```python
from build123d import *

# Parameters (mm, degrees)
SKETCH1_W           = 149
SKETCH1_H           = 168
SKETCH1_W_2         = 125
SKETCH1_H_2         = 144
BOSS_EXTRUDE1_DEPTH = 7
FILLET1_R           = 5
FILLET2_R           = 5
FILLET3_R           = 5
FILLET4_R           = 5
CUT_EXTRUDE1_DEPTH  = 3
SKETCH6_R           = 1.325
CUT_EXTRUDE2_DEPTH  = 4
CUT_EXTRUDE3_DEPTH  = 2


with BuildPart() as part:
    # Sketch1 → Boss-Extrude1 (new body)
    with BuildSketch(Plane(origin=(0, 0, 0), x_dir=(1, 0, 0), z_dir=(0, 1, 0))):
        with Locations((-8.812010444, -5.018276762)):
            Rectangle(SKETCH1_W, SKETCH1_H)
        with Locations((-8.812010444, -5.018276762)):
            Rectangle(SKETCH1_W_2, SKETCH1_H_2, mode=Mode.SUBTRACT)
    extrude(amount=BOSS_EXTRUDE1_DEPTH)

    # Fillet1
    fillet1_edges = [part.edges().sort_by_distance(p)[0] for p in [
        (65.687989556, 3.5, 89.018276762),
    ]]
    fillet(fillet1_edges, radius=FILLET1_R)

    # Fillet2
    fillet2_edges = [part.edges().sort_by_distance(p)[0] for p in [
        (-83.312010444, 3.5, 89.018276762),
    ]]
    fillet(fillet2_edges, radius=FILLET2_R)

    # Fillet3
    fillet3_edges = [part.edges().sort_by_distance(p)[0] for p in [
        (-83.312010444, 3.5, -78.981723238),
    ]]
    fillet(fillet3_edges, radius=FILLET3_R)

    # Fillet4
    fillet4_edges = [part.edges().sort_by_distance(p)[0] for p in [
        (65.687989556, 3.5, -78.981723238),
    ]]
    fillet(fillet4_edges, radius=FILLET4_R)

    # Sketch4 → Cut-Extrude1 (cut)
    with BuildSketch(Plane.XZ):
        Polygon((-40.312010444, 80.018276762), (-25.812010444, 80.018276762), (-25.812010444, 84.518276762), (-60.812010444, 84.518276762), (-60.812010444, 80.018276762), (-46.312010444, 80.018276762), (-46.312010444, 77.018276762), (-40.312010444, 77.018276762), align=None)
        Polygon((22.687989556, 77.018276762), (22.687989556, 80.018276762), (8.187989556, 80.018276762), (8.187989556, 84.518276762), (43.187989556, 84.518276762), (43.187989556, 80.018276762), (28.687989556, 80.018276762), (28.687989556, 77.018276762), align=None)
        Polygon((53.687989556, 47.018276762), (56.687989556, 47.018276762), (56.687989556, 66.518276762), (61.187989556, 66.518276762), (61.187989556, 21.518276762), (56.687989556, 21.518276762), (56.687989556, 41.018276762), (53.687989556, 41.018276762), align=None)
        Polygon((53.687989556, -35.981723238), (56.687989556, -35.981723238), (56.687989556, -13.981723238), (61.187989556, -13.981723238), (61.187989556, -63.981723238), (56.687989556, -63.981723238), (56.687989556, -41.981723238), (53.687989556, -41.981723238), align=None)
        Polygon((43.187989556, -69.981723238), (43.187989556, -74.481723238), (8.187989556, -74.481723238), (8.187989556, -69.981723238), (22.687989556, -69.981723238), (22.687989556, -66.981723238), (28.687989556, -66.981723238), (28.687989556, -69.981723238), align=None)
        Polygon((-40.312010444, -66.981723238), (-40.312010444, -69.981723238), (-25.812010444, -69.981723238), (-25.812010444, -74.481723238), (-60.812010444, -74.481723238), (-60.812010444, -69.981723238), (-46.312010444, -69.981723238), (-46.312010444, -66.981723238), align=None)
        Polygon((-71.312010444, -41.981723238), (-74.312010444, -41.981723238), (-74.312010444, -63.981723238), (-78.812010444, -63.981723238), (-78.812010444, -13.981723238), (-74.312010444, -13.981723238), (-74.312010444, -35.981723238), (-71.312010444, -35.981723238), align=None)
        Polygon((-71.312010444, 41.018276762), (-74.312010444, 41.018276762), (-74.312010444, 21.518276762), (-78.812010444, 21.518276762), (-78.812010444, 66.518276762), (-74.312010444, 66.518276762), (-74.312010444, 47.018276762), (-71.312010444, 47.018276762), align=None)
    extrude(amount=-CUT_EXTRUDE1_DEPTH, mode=Mode.SUBTRACT)

    # Sketch6 → Cut-Extrude2 (cut)
    with BuildSketch(Plane.XZ):
        with Locations(Location((-76.579777397, 82.286043715, 0), (0, 0, 270))):
            Circle(SKETCH6_R)
        with Locations(Location((58.955756509, 82.286043715, 0), (0, 0, 270))):
            Circle(SKETCH6_R)
        with Locations(Location((58.955756509, -72.249490191, 0), (0, 0, 270))):
            Circle(SKETCH6_R)
        with Locations(Location((-76.579777397, -72.249490191, 0), (0, 0, 270))):
            Circle(SKETCH6_R)
    extrude(amount=-CUT_EXTRUDE2_DEPTH, mode=Mode.SUBTRACT)

    # Sketch7 → Cut-Extrude3 (cut)
    with BuildSketch(Plane.XZ.offset(-3)):
        Polygon((53.687989556, -35.981723238), (56.687989556, -35.981723238), (56.687989556, -30.981723238), (61.187989556, -30.981723238), (61.187989556, -46.981723238), (56.687989556, -46.981723238), (56.687989556, -41.981723238), (53.687989556, -41.981723238), align=None)
        Polygon((53.687989556, 47.018276762), (56.687989556, 47.018276762), (56.687989556, 52.018276762), (61.187989556, 52.018276762), (61.187989556, 36.018276762), (56.687989556, 36.018276762), (56.687989556, 41.018276762), (53.687989556, 41.018276762), align=None)
        Polygon((28.687989556, 77.018276762), (28.687989556, 80.018276762), (33.687989556, 80.018276762), (33.687989556, 84.518276762), (17.687989556, 84.518276762), (17.687989556, 80.018276762), (22.687989556, 80.018276762), (22.687989556, 77.018276762), align=None)
        Polygon((-40.312010444, 77.018276762), (-40.312010444, 80.018276762), (-35.312010444, 80.018276762), (-35.312010444, 84.518276762), (-51.312010444, 84.518276762), (-51.312010444, 80.018276762), (-46.312010444, 80.018276762), (-46.312010444, 77.018276762), align=None)
        Polygon((-71.312010444, 47.018276762), (-74.312010444, 47.018276762), (-74.312010444, 52.018276762), (-78.812010444, 52.018276762), (-78.812010444, 36.018276762), (-74.312010444, 36.018276762), (-74.312010444, 41.018276762), (-71.312010444, 41.018276762), align=None)
        Polygon((-71.312010444, -35.981723238), (-74.312010444, -35.981723238), (-74.312010444, -30.981723238), (-78.812010444, -30.981723238), (-78.812010444, -46.981723238), (-74.312010444, -46.981723238), (-74.312010444, -41.981723238), (-71.312010444, -41.981723238), align=None)
        Polygon((-46.312010444, -66.981723238), (-46.312010444, -69.981723238), (-51.312010444, -69.981723238), (-51.312010444, -74.481723238), (-35.312010444, -74.481723238), (-35.312010444, -69.981723238), (-40.312010444, -69.981723238), (-40.312010444, -66.981723238), align=None)
        Polygon((22.687989556, -66.981723238), (22.687989556, -69.981723238), (17.687989556, -69.981723238), (17.687989556, -74.481723238), (33.687989556, -74.481723238), (33.687989556, -69.981723238), (28.687989556, -69.981723238), (28.687989556, -66.981723238), align=None)
    extrude(amount=-CUT_EXTRUDE3_DEPTH, mode=Mode.SUBTRACT)


solid = part.part
```
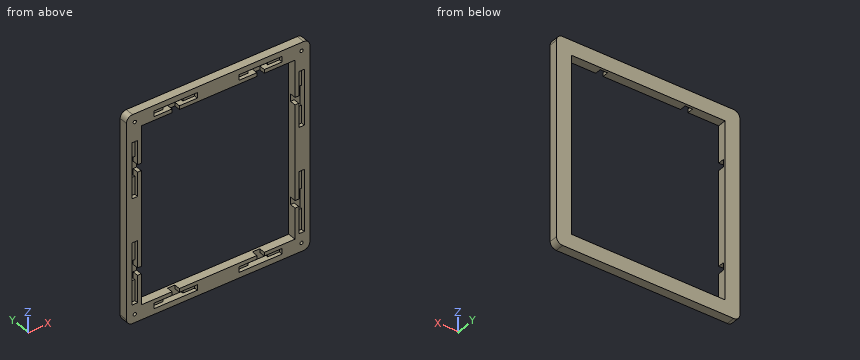
The model under review builds one solid part; all positions refer to its coordinate system, in mm. Coordinates: 2 decimals unless noted, no trailing zeros. Write each loop counter-clockwise with the first axis right and the second up, starting at its lowest first coordinate (ties: lowest second). Pieces come first, ordered by that corner, then holes.
1) We need section B-B on x = -28. State the section outline as (y, z) points.
2) We need section C-C on z = -4. State the section outline as (x, y) points.
3) We need section A-A on z = 39. State the section outline as (x, y) points, then the cut area to 3 significant figures.
4) We need section D-D on x = -5. State the section outline as (y, z) points, then the cut area to 3 significant figures.
5) To check wall thickness, follow probe 1 along Z at (x, y) = (-48, 4); probe 2 along X at (y, z) = (1, -20.5); probe 3 along X at (y, z) = (3.5, 1.5). State the ranges of each line that lie inside material, in increasing order.
Answer list:
1. outline: (0, -78.98) - (7, -78.98) - (7, -66.98) - (0, -66.98) - (0, -69.98) - (3, -69.98) - (3, -74.48) - (0, -74.48) - close; (0, 77.02) - (7, 77.02) - (7, 89.02) - (0, 89.02) - (0, 84.52) - (3, 84.52) - (3, 80.02) - (0, 80.02) - close
2. outline: (-83.31, 0) - (-71.31, 0) - (-71.31, 7) - (-83.31, 7) - close; (53.69, 0) - (65.69, 0) - (65.69, 7) - (53.69, 7) - close
3. outline: (-83.31, 0) - (-78.81, 0) - (-78.81, 5) - (-74.31, 5) - (-74.31, 0) - (-71.31, 0) - (-71.31, 7) - (-83.31, 7) - close; (53.69, 0) - (56.69, 0) - (56.69, 5) - (61.19, 5) - (61.19, 0) - (65.69, 0) - (65.69, 7) - (53.69, 7) - close
3. area: 123 mm2
4. outline: (0, -78.98) - (7, -78.98) - (7, -66.98) - (0, -66.98) - close; (0, 77.02) - (7, 77.02) - (7, 89.02) - (0, 89.02) - close
4. area: 168 mm2
5. probe 1: z = -78.98 to -74.48, -69.98 to -66.98, 77.02 to 80.02, 84.52 to 89.02
5. probe 2: x = -83.31 to -78.81, -74.31 to -71.31, 53.69 to 56.69, 61.19 to 65.69
5. probe 3: x = -83.31 to -71.31, 53.69 to 65.69
